Study the drawing (mm; zero at the part's minimum x, y, z) and answer. A direction names the side the tool comes from. Round coordinates to 2 decimals unless told otherwise and drop trailing zeros. Order: outer loops, then holes, each group sorted by start corner. A loop starts at its lowest first (then second) coordinate and runs counter-clockwise, first axis right, second up. Notation, with made-up numbers: (23, -5) - (33, -5) arc R15 cw to (33, 18) - close; hole circle Ø6 at (13, -7). An arc over 180 degrees is marked (long way). Put each result on its own line as item: value.
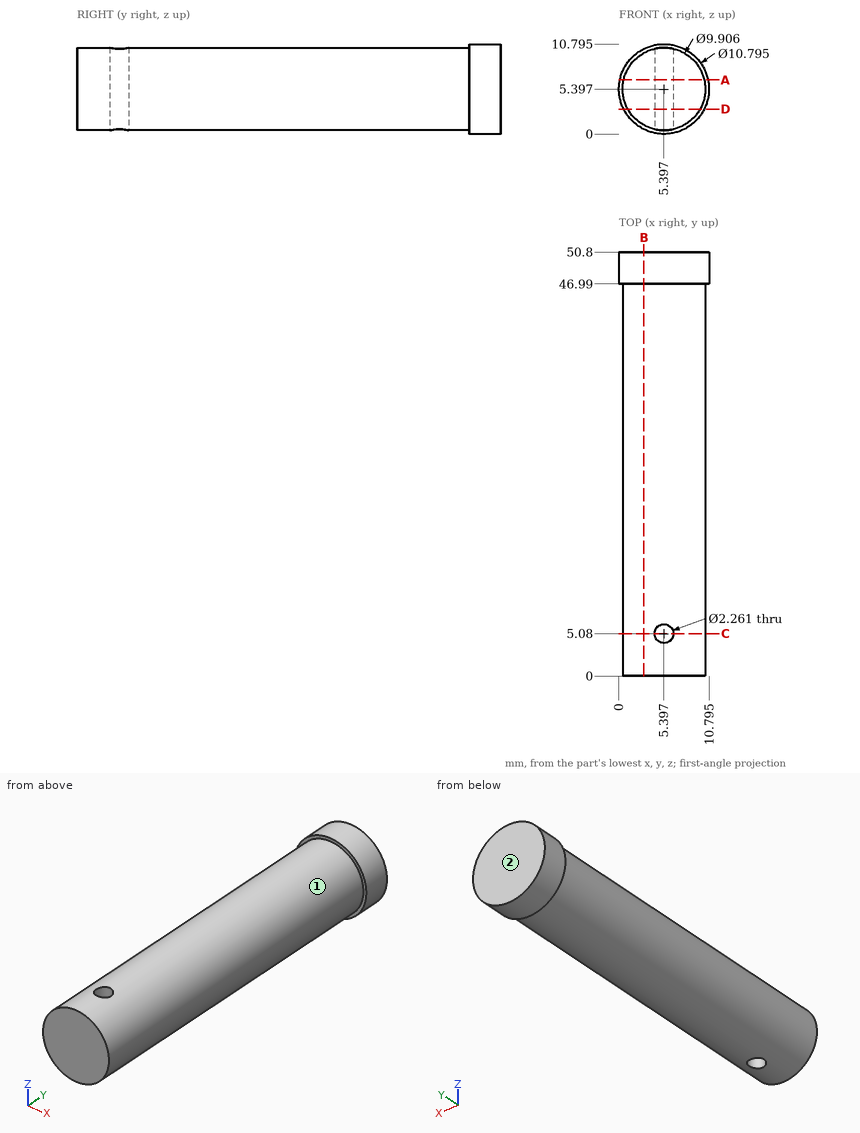
1) Given pin 1 Ø1.5 at (x, y) = (7.5, 31) entering from +Z; pin 2 Ø1.5 at (y, z) = (7.5, 9) entering from +X; pin 3 Ø1.5 at (y, z) = (8.5, 6) entering from -X (1 decimal), each flat-ended and moving along its own axis, determine where each tip first touches the part or whether it passes through.
Findings below:
pin 1: stops at z = 10.16
pin 2: stops at x = 9.45
pin 3: stops at x = 0.4
2) A cutting plane is placed at D-D on z = 3. Write down the section's boundary in (x, y), then the cut area to 3 significant figures.
Findings below:
outline: (0.56, 46.99) - (1.06, 46.99) - (1.06, 0) - (9.73, 0) - (9.73, 46.99) - (10.23, 46.99) - (10.23, 50.8) - (0.56, 50.8) - close; hole circle Ø2.26 at (5.4, 5.08)
area: 440 mm2
3) A cutting plane is placed at C-C on y = 5.08. Write down the section's boundary in (x, z) (1 decimal).
Findings below:
outline: (4.3, 0.6) - (4.3, 10.2) arc R5 ccw to start; (6.5, 0.6) arc R5 ccw to (6.5, 10.2) - close
4) A cutting plane is placed at B-B on x = 3. Write down the section's boundary in (y, z), then the cut area to 3 significant figures.
Findings below:
outline: (0, 1.06) - (46.99, 1.06) - (46.99, 0.56) - (50.8, 0.56) - (50.8, 10.23) - (46.99, 10.23) - (46.99, 9.73) - (0, 9.73) - close
area: 444 mm2
5) Straight lines are drawn through the part: L1, parallel to Y at x = 5.5, z = 3.25 (1 decimal); L2, parallel to Y at x = 2.5, z = 1; L3, parallel to Y at x = 4.5, z = 7.5 (1 decimal). For each, find the intervals that lie inside material, in ascending order. Write a range as from..to.
Findings below:
L1: y = 0..4, 6.2..50.8
L2: y = 46.99..50.8
L3: y = 0..4.4, 5.8..50.8
6) For the marked faces 1 and 2, determine the directions among +Z, -Z, +X, -X, +Y, -Y from which every point of the face is accessible in a straight line to the end or side of a thin tool.
Findings below:
face 1: -Y
face 2: +Z, -Z, +X, -X, +Y
7) A cutting plane is placed at A-A on z = 6.5. Write down the section's boundary in (x, y), then the cut area to 3 significant figures.
Findings below:
outline: (0.11, 46.99) - (0.57, 46.99) - (0.57, 0) - (10.23, 0) - (10.23, 46.99) - (10.68, 46.99) - (10.68, 50.8) - (0.11, 50.8) - close; hole circle Ø2.26 at (5.4, 5.08)
area: 490 mm2
